Verification items for the finished model (mm, model axes). Round coordinates to 2 decimals unless told otherwise and drop trailing zeros. Write each loop counter-clockwise with the first axis right and the second up, starting at its lowest first coordinate (ties: lowest second). Pieces come first, ordered by that corner, then holes. Notation, with made-up numbers: M 85,13 L 139,13 A22 ccw 139,28 Z; hole C -7.5,-25.5 d6. An arc over 180 degrees is marked long. Write each question's results on one line, items separated by ' | '.
from build123d import *

# Parameters (mm, degrees)
EXTRUDE_1_4_DEPTH = 3.1
SKETCH4_R         = 2
M4_DRILL_DEPTH    = 8
SKETCH5_R         = 2
M4_DRILL2_DEPTH   = 8
SKETCH6_R         = 2.25
M4_THROUGH_DEPTH  = 6.2


with BuildPart() as part:
    # Sketch1 → 1/4 (new, symmetric)
    with BuildSketch(Plane.XY):
        Polygon((-20, 45), (20, 45), (30, 10), (30, -45), (-30, -45), (-30, 10), align=None)
    extrude(amount=EXTRUDE_1_4_DEPTH, both=True)

    # Sketch4 → M4_DRILL (cut)
    with BuildSketch(Plane(origin=(0, 45, 0), x_dir=(1, 0, 0), z_dir=(0, 1, 0))):
        with Locations(Location((-12, 0, 0), (0, 0, 180))):
            Circle(SKETCH4_R)
        with Locations((12, 0)):
            Circle(SKETCH4_R)
    extrude(amount=-M4_DRILL_DEPTH, mode=Mode.SUBTRACT)

    # Sketch5 → M4_DRILL2 (cut)
    with BuildSketch(Plane(origin=(0, -45, 0), x_dir=(-1, 0, 0), z_dir=(0, -1, 0))):
        with Locations(Location((-20, 0, 0), (0, 0, 180))):
            Circle(SKETCH5_R)
        with Locations((20, 0)):
            Circle(SKETCH5_R)
        with Locations(Location((0, 0, 0), (0, 0, 180))):
            Circle(SKETCH5_R)
    extrude(amount=-M4_DRILL2_DEPTH, mode=Mode.SUBTRACT)

    # Sketch6 → M4_through (cut)
    with BuildSketch(Plane.XY.offset(3.1)):
        with Locations((-25.2375, -31)):
            Circle(SKETCH6_R)
        with Locations((25.2375, -31)):
            Circle(SKETCH6_R)
        with Locations((-15.2375, 31)):
            Circle(SKETCH6_R)
        with Locations((15.2375, 31)):
            Circle(SKETCH6_R)
    extrude(amount=-M4_THROUGH_DEPTH, mode=Mode.SUBTRACT)


solid = part.part
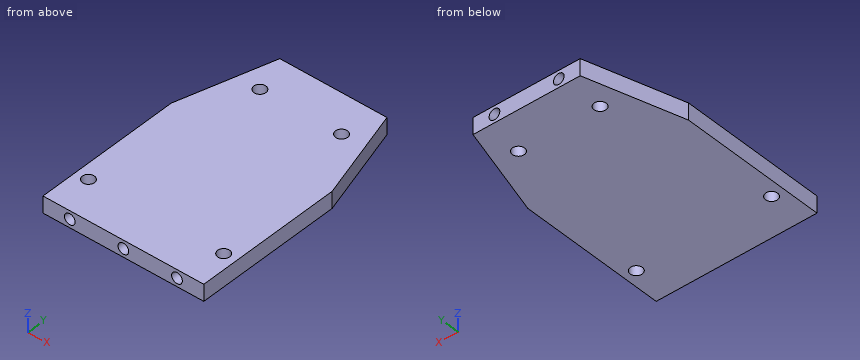
1) Sectioned sample at C-C, the plane x = 0. Record the cut outline in (y, z).
Calculated:
outline: M -45,-3.1 L 45,-3.1 L 45,3.1 L -45,3.1 L -45,2 L -37,2 L -37,-2 L -45,-2 Z
2) Sectioned sample at A-A, the plane z = 0. Count the separate pieces of the cut face and the enclosed holes in it, and give its area (3 significant figures).
Calculated:
separate pieces: 1 | enclosed holes: 4 | area: 4,830 mm²
3) Material ranges on line 1 (Z direction, x = 20, y = -39); line 2 (Y direction, x = 11.5, z = 1.25); line 3 (Y direction, x = 17, z = -1.75), recorded low to high. Write a range as [from, to].
Calculated:
line 1: z = [-3.1, -2], [2, 3.1] | line 2: y = [-45, 37] | line 3: y = [-45, 29.6], [32.4, 45]
4) Sectioned sample at D-D, the plane x = -25. Record the cut outline in (y, z).
Calculated:
outline: M -45,-3.1 L -33.24,-3.1 L -33.24,3.1 L -45,3.1 Z; M -28.76,-3.1 L 27.5,-3.1 L 27.5,3.1 L -28.76,3.1 Z
5) Sectioned sample at B-B, the plane y = -31. Record the cut outline in (x, z), and give its area (3 significant figures).
Calculated:
outline: M -30,-3.1 L -27.49,-3.1 L -27.49,3.1 L -30,3.1 Z; M -22.99,-3.1 L 22.99,-3.1 L 22.99,3.1 L -22.99,3.1 Z; M 27.49,-3.1 L 30,-3.1 L 30,3.1 L 27.49,3.1 Z | area: 316 mm²
6) Depth check by flat-ended pin: P1, Ø2, axis at x = 12.5, z = 0.5, coming from the +Y side; P2, Ø5, axis at x = 25.24, y = -31, coming from the +Z side; P3, Ø3, axis at x = 0, z = 0, coming from the -Y side; P4, Ø2.5, axis at x = -15.24, y = 31, coming from the -Z side. Enter the tip coordinate at first touch or a pass-through.
Calculated:
P1: stops at y = 37 | P2: stops at z = 3.1 | P3: stops at y = -37 | P4: passes through
